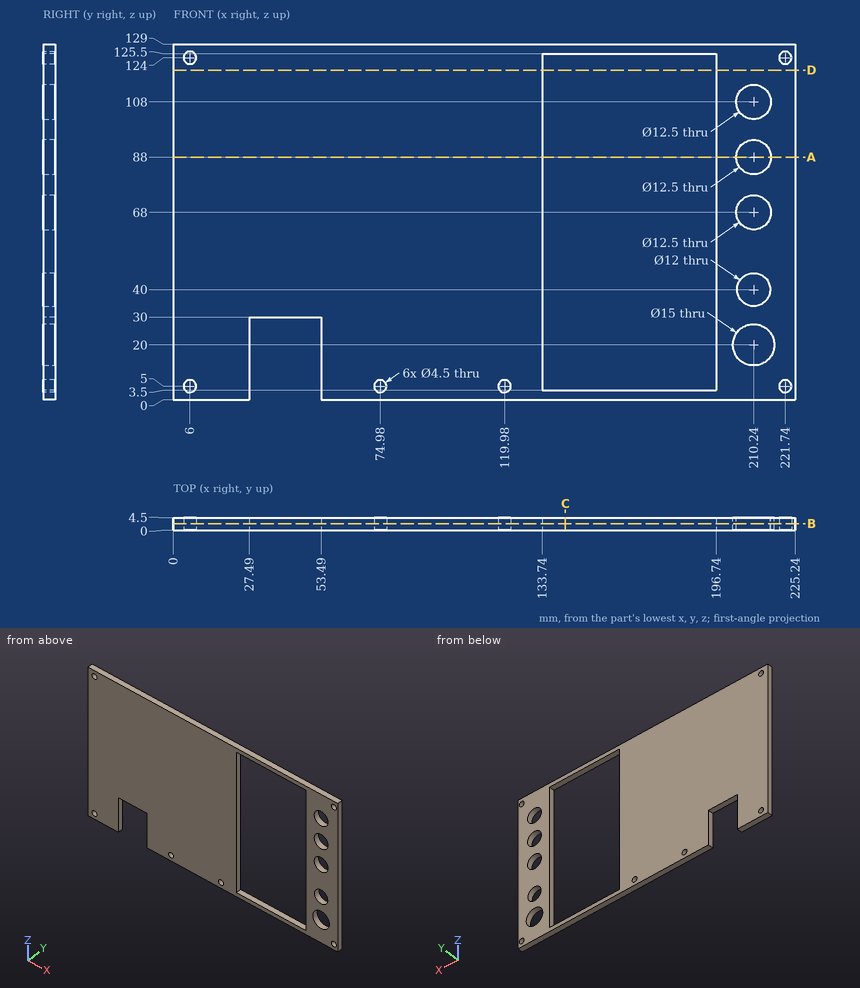
Geometry check sheet. Reference: drawing and pictorial views, mm from the part's lowest x, y, z. Give positions to 0.01 mm unless a question says otherwise; leave off trailing zeros. Loops run counter-clockwise (first coordinate to the right, second up) from the corner with the lowest first, then second, coordinate; pieces in that order, holes last. Notation, with made-up numbers: (-31.75, 80) - (23.25, 80) arc R13 ccw to (23.25, 89) - close; hole circle Ø2 at (-11, 54). An arc over 180 degrees is marked (long way). One line per question, with ' | ' between items. Start each with the question number.
1. Cross-section at A-A, the plane z = 88. Enter the section's corners in (x, y), plus the area to 3 significant figures.
2. Cross-section at B-B, the plane y = 2.45. Give the number of separate pieces and of enclosed holes in the cut face, plus the area to 3 significant figures.
3. Material ranges on line 1 along Z through (x, y) = (221.74, 1); line 2 along X through (y, z) = (2, 108); line 3 along X through (y, z) = (2.8, 78), recorded low to high. Write a range as [from, to].
4. Cross-section at D-D, the plane z = 119.5. Enter the section's corners in (x, y), plus the area to 3 significant figures.
5. Gauge pin test, flat ends, axial feed: pin 1 Ø2.5 at (x, z) = (74.98, 5) entering from -Y; pin 2 Ø1.3 at (x, y) = (160, 3) entering from -Z. Record the tip position at first contact, or that the pin passes through.
6. Cross-section at C-C, the plane x = 142. Enter the section's corners in (y, z), plus the area to 3 significant figures.
Check result:
1) outline: (0, 0) - (133.74, 0) - (133.74, 4.5) - (0, 4.5) - close; (196.74, 0) - (203.99, 0) - (203.99, 4.5) - (196.74, 4.5) - close; (216.49, 0) - (225.24, 0) - (225.24, 4.5) - (216.49, 4.5) - close | area: 674 mm2
2) separate pieces: 1 | enclosed holes: 12 | area: 19,800 mm2
3) line 1: z = [0, 2.75], [7.25, 121.75], [126.25, 129] | line 2: x = [0, 133.74], [196.74, 203.99], [216.49, 225.24] | line 3: x = [0, 133.74], [196.74, 225.24]
4) outline: (0, 0) - (133.74, 0) - (133.74, 4.5) - (0, 4.5) - close; (196.74, 0) - (225.24, 0) - (225.24, 4.5) - (196.74, 4.5) - close | area: 730 mm2
5) pin 1: passes through | pin 2: stops at z = 0
6) outline: (0, 0) - (4.5, 0) - (4.5, 3.5) - (0, 3.5) - close; (0, 125.5) - (4.5, 125.5) - (4.5, 129) - (0, 129) - close | area: 31.5 mm2
